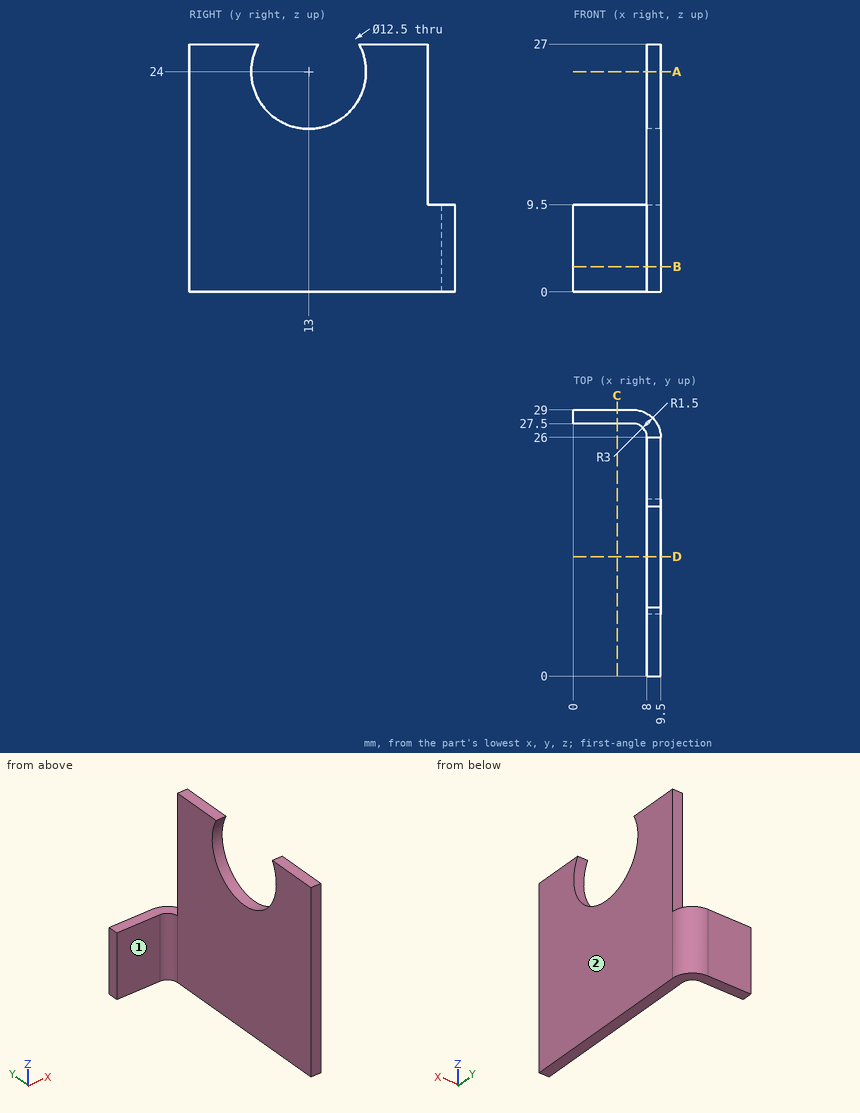
Geometry check sheet. Reference: drawing and pictorial views, mm from the part's lowest x, y, z. A direction names the side the tool comes from. Round coordinates to 2 decimals unless told otherwise and drop trailing zeros. Loops run counter-clockwise (first coordinate to the right, second up) from the corner with the lowest first, then second, coordinate; pieces in that order, holes last. Notation, with made-up numbers: M 17,23 L 57,23 A23 cw 57,53 Z; hole C 37.5,-6.5 d11. An arc over 180 degrees is marked long. Return JSON: item names as keys, results as strings. Group by question number.
(1) Scan lines: line 1 along Y through (x, z) = (9.15, 24); line 2 along Y through (x, z) = (2.5, 1.5); line 3 along X through (y, z) = (7.5, 13). Record each from-to range of solid material in increasing order. Write a range as [from, to].
(2) Section check C-C, the plane x = 4.75. Enter the section's corners in (y, z).
(3) Go/stop test with flat-tipped pins: pin 1 (1.6 mm diameter, centred on x = 9, z = 21.5, fed in from +Y); pin 2 (2.5 mm diameter, centred on x = 3, y = 27, fed in from +Z); pin 3 (2 mm diameter, centred on x = 2, z = 6, fed in from -Y). Record where each tip stops, or that it passes through.
(4) Section check D-D, the plane y = 13. Enter the section's corners in (x, z).
(5) Section check A-A, the plane z = 24. Enter the section's corners in (x, y), and give its area (4 significant figures).
(6) Set-up check for the marked faces 1 and 2: record each of +Z, -Z, +X, -X, +Y, -Y from which the full face is reachable in a straight line by a thin tool's end or side.
(7) Section check B-B, the plane z = 2.75. Enter the section's corners in (x, y), and give its area (3 significant figures).
Data:
{
 "1": {"line 1": "[0, 6.75], [19.25, 26]", "line 2": "[27.5, 29]", "line 3": "[8, 9.5]"},
 "2": {"outline": "M 27.5,0 L 29,0 L 29,9.5 L 27.5,9.5 Z"},
 "3": {"pin 1": "y = 26", "pin 2": "z = 9.5", "pin 3": "y = 27.5"},
 "4": {"outline": "M 8,0 L 9.5,0 L 9.5,17.75 L 8,17.75 Z"},
 "5": {"outline": "M 8,0 L 9.5,0 L 9.5,6.75 L 8,6.75 Z; M 8,19.25 L 9.5,19.25 L 9.5,26 L 8,26 Z", "area": "20.25 mm²"},
 "6": {"face 1": "+Z, -Z, -X, -Y", "face 2": "+Z, -Z, +X, +Y, -Y"},
 "7": {"outline": "M 0,27.5 L 6.5,27.5 A1.5 cw 8,26 L 8,0 L 9.5,0 L 9.5,26 A3 ccw 6.5,29 L 0,29 Z", "area": "54.1 mm²"}
}
